The listing builds one solid part. Answer for the finished solid, in the listing's coordinates (mm). Face numbers are marked on the shaded views. A direction names the side the tool comes from. Coordinates: 2 decimals unless noted, no trailing zeros. Write each loop counter-clockwise with the first axis right and the second up, starting at its lowest first coordinate (ties: lowest second). Pieces come first, ordered by that corner, then holes. Notation, with made-up numbers: M 70.5,88 L 76.5,88 A24 ccw 76.5,121 Z; hole C 86.25,41.5 d6. An arc over 180 degrees is marked long. Answer as CSV lines item,"result". Start each with the question number.
```python
from build123d import *

# Parameters (mm, degrees)
BOSS_EXTRUDE1_DEPTH = 40
SHELL1_T            = 4
SKETCH2_W           = 38
SKETCH2_H           = 8
CUT_EXTRUDE1_DEPTH  = 50.505693367
BOSS_EXTRUDE2_DEPTH = 40
SKETCH4_R           = 2.1
CUT_EXTRUDE2_DEPTH  = 57.708559772
SKETCH5_R           = 4
CUT_EXTRUDE4_DEPTH  = 28
LPATTERN1_COUNT     = 2
LPATTERN1_PITCH     = 22
FILLET1_R           = 3


with BuildPart() as part:
    # Sketch1 → Boss-Extrude1 (new body)
    with BuildSketch(Plane.XY):
        with BuildLine():
            Line((-15.770198569, -12.053486897), (14.229801431, -12.053486897))
            Line((14.229801431, -12.053486897), (14.229801431, -8.053486897))
            Line((14.229801431, -8.053486897), (6.229801431, -8.053486897))
            Line((6.229801431, -8.053486897), (6.229801431, -2.053486897))
            Line((6.229801431, -2.053486897), (2.31145028, 5.223450953))
            ThreePointArc((2.31145028, 5.223450953), (-0.770198569, 17.446513103), (-3.851847419, 5.223450953))
            Line((-3.851847419, 5.223450953), (-7.770198569, -2.053486897))
            Line((-7.770198569, -2.053486897), (-7.770198569, -8.053486897))
            Line((-7.770198569, -8.053486897), (-15.770198569, -8.053486897))
            Line((-15.770198569, -8.053486897), (-15.770198569, -12.053486897))
        make_face()
    extrude(amount=BOSS_EXTRUDE1_DEPTH)

    # Shell1
    shell1_openings = [part.faces().sort_by_distance(p)[0] for p in [
        (-0.770198569, -0.27560318, 0),
        (-0.770198569, -0.27560318, 40),
    ]]
    offset(amount=SHELL1_T, openings=shell1_openings, kind=Kind.INTERSECTION)

    # Sketch2 → Cut-Extrude1 (cut, through all)
    with BuildSketch(Plane.XY.offset(40)):
        with Locations((-0.770198569, -12.053486897)):
            Rectangle(SKETCH2_W, SKETCH2_H)
    extrude(amount=-CUT_EXTRUDE1_DEPTH, mode=Mode.SUBTRACT)

    # Sketch3 → Boss-Extrude2 (add, through all)
    with BuildSketch(Plane.XY.offset(40)):
        Polygon((-19.770198569, 26.946513103), (18.229801431, 26.946513103), (18.229801431, -8.053486897), (6.229801431, -8.053486897), (6.229801431, 17.511933237), (-7.770198569, 17.511933237), (-7.770198569, -8.053486897), (-19.770198569, -8.053486897), align=None)
    extrude(amount=-BOSS_EXTRUDE2_DEPTH)

    # Sketch4 → Cut-Extrude2 (cut, through all)
    with BuildSketch(Plane.XZ.offset(8.053486897)):
        with Locations(Location((-11.770198569, 20, 0), (0, 0, 270))):
            Circle(SKETCH4_R)
    cut_extrude2 = extrude(amount=-CUT_EXTRUDE2_DEPTH, mode=Mode.SUBTRACT)

    # Sketch5 → Cut-Extrude4 (cut)
    with BuildSketch(Plane(origin=(0, 26.946513103, 0), x_dir=(1, 0, 0), z_dir=(0, 1, 0))):
        with Locations(Location((-11.770198569, -20, 0), (0, 0, 270))):
            Circle(SKETCH5_R)
    cut_extrude4 = extrude(amount=-CUT_EXTRUDE4_DEPTH, mode=Mode.SUBTRACT)

    # LPattern1: Cut-Extrude2, Cut-Extrude4 ×2
    with Locations(*[(i * LPATTERN1_PITCH, 0, 0) for i in range(1, LPATTERN1_COUNT)]):
        add(cut_extrude2, mode=Mode.SUBTRACT)
        add(cut_extrude4, mode=Mode.SUBTRACT)

    # Fillet1
    fillet1_edges = [part.edges().sort_by_distance(p)[0] for p in [
        (-0.770198569, 26.946513103, 40),
        (-19.770198569, 26.946513103, 20),
        (18.229801431, 26.946513103, 20),
        (-0.770198569, 26.946513103, 0),
        (-19.770198569, 9.446513103, 0),
        (-19.770198569, 9.446513103, 40),
        (18.229801431, 9.446513103, 0),
        (18.229801431, 9.446513103, 40),
    ]]
    fillet(fillet1_edges, radius=FILLET1_R)


solid = part.part
```
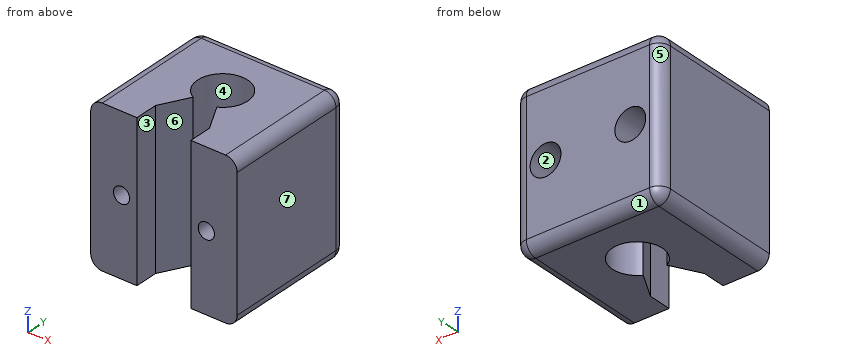
1) The part is cut by section A-A (z = 20). Determine the outline of the cut face in (x, y).
2) For a pull along Y with two mould halves and no side action, classify the marked faces 4, 5, 6 and 7 as +Y half, -Y half, draft (parallel to the pull), parting line (faces both ways), or undercut.
3) The part is cut by section C-C (z = 31.5). Determine the outline of the cut face in (x, y), then the cut area to 3 significant figures.
4) Find the intervals of material crossed by line 1 (X direction, y = -4, z = 20); line 2 (X direction, y = -2, z = 20); line 3 (Z direction, x = 10, y = 9.5), in increasing order. Write a range as from..to.
5) Each of these flat-tipped pins is pushed along its axis until it touches: P1, Ø10, axis at x = -1, z = 6.5, coming from the -Y side; P2, Ø5, axis at x = -5, y = 9, coming from the -Z side; P3, Ø4, axis at x = 10, z = 21, coming from the +Y side. Where does it stop, or does it pass through?
6) Which of the six approach directions +Z, -Z, +X, -X, +Y, -Y give full straight-line access (tool end or side, diameter ignored) to the marked faces 1, 2 and 3?
7) The part is cut by section D-D (x = 5). Determine the outline of the cut face in (y, z), then the cut area to 3 significant figures.
8) The part is cut by section B-B (y = 8). Determine the outline of the cut face in (x, z).
Completed:
1,outline,"M -19.77,-8.05 L -13.87,-8.05 L -13.87,-1.05 L -15.77,-1.05 L -15.77,26.95 L -16.77,26.95 A3 ccw -19.77,23.95 Z; M -9.67,-8.05 L -7.77,-8.05 L -7.77,-2.05 L -3.85,5.22 A6.5 cw long 2.31,5.22 L 6.23,-2.05 L 6.23,-8.05 L 8.13,-8.05 L 8.13,-1.05 L 6.23,-1.05 L 6.23,26.95 L -7.77,26.95 L -7.77,-1.05 L -9.67,-1.05 Z; M 12.33,-8.05 L 18.23,-8.05 L 18.23,23.95 A3 ccw 15.23,26.95 L 14.23,26.95 L 14.23,-1.05 L 12.33,-1.05 Z"
2,face 4,"undercut"
2,face 5,"+Y half"
2,face 6,"-Y half"
2,face 7,"draft"
3,outline,"M -19.77,-8.05 L -7.77,-8.05 L -7.77,-2.05 L -3.85,5.22 A6.5 cw long 2.31,5.22 L 6.23,-2.05 L 6.23,-8.05 L 18.23,-8.05 L 18.23,23.95 A3 ccw 15.23,26.95 L -16.77,26.95 A3 ccw -19.77,23.95 Z"
3,area,"1,040 mm²"
4,line 1,"-19.77..-13.87, -9.67..-7.77, 6.23..8.13, 12.33..18.23"
4,line 2,"-19.77..-13.87, -9.67..-7.74, 6.2..8.13, 12.33..18.23"
4,line 3,"0..16.01, 23.99..40"
5,P1,"y = 1.23"
5,P2,"z = 0"
5,P3,"y = -1.05"
6,face 1,"-Z, +X, -X, +Y"
6,face 2,"+Y"
6,face 3,"+Z, -Z, -Y"
7,outline,"M 0.23,0 L 7.95,0 L 7.95,40 L 0.23,40 Z; M 13.94,0 L 23.95,0 A3 ccw 26.95,3 L 26.95,37 A3 ccw 23.95,40 L 13.94,40 Z"
7,area,"825 mm²"
8,outline,"M -19.77,3 A3 ccw -16.77,0 L -6.56,0 L -6.56,40 L -16.77,40 A3 ccw -19.77,37 Z; M 5.02,0 L 15.23,0 A3 ccw 18.23,3 L 18.23,37 A3 ccw 15.23,40 L 5.02,40 Z; hole C -11.77,20 d8; hole C 10.23,20 d8"
